Source: CAD feature listing. Evaluate the final solid. Frame: model axes, mm. A direction names the side the tool comes from. Round coordinates to 2 decimals unless told otherwise and drop trailing zeros. Write each loop counter-clockwise with the first axis right and the second up, starting at its lowest first coordinate (ties: lowest second). Pieces come first, ordered by that corner, then holes.
from build123d import *

# Parameters (mm, degrees)
F1_DEPTH    = 2.25
F2_R        = 10.9
F3_DEPTH    = 10.6
F5_DEPTH    = 9.5
F6_T2_ANGLE = 290.6956436441
F6_T4_ANGLE = 110.5630137602
F7_R        = 8.6
F8_DEPTH    = 10
F9_R        = 7.38
F10_DEPTH   = 7
F11_R       = 10.9
F11_R_2     = 9.6734059383
F12_DEPTH   = 8
F13_R       = 9.5
F14_DEPTH   = 1


# Not quite as in the source:
# - a fillet or chamfer that OpenCascade refuses, or shapes differently, is made with other operations: its cross-section is extruded or revolved along the edge and cut away or added


with BuildPart() as f1:
    # F0 (on Top) → F1 (new body)
    with BuildSketch(Plane.XY):
        Polygon((0, 9), (9, 0), (23, 0), (32, 9), (32, 23), (23, 32), (9, 32), (0, 23), align=None)
    extrude(amount=F1_DEPTH)

    # F2 (on Top) → F3 (join)
    with BuildSketch(Plane.XY):
        with Locations((16, 16)):
            Circle(F2_R)
    extrude(amount=F3_DEPTH)

    # F4 (on face) → F5 (join)
    with BuildSketch(Plane(origin=(0, 0, 0), x_dir=(1, 0, 0), z_dir=(0, 0, -1))):
        with BuildLine():
            ThreePointArc((10.8502427242, -6.45), (10.4390813008, -25.3165810908), (26.85, -16))
            ThreePointArc((26.85, -16), (25.3165810908, -10.4390813008), (21.1497572758, -6.45))
            Line((21.1497572758, -6.45), (10.8502427242, -6.45))
        make_face()
    extrude(amount=F5_DEPTH)

    # F6: chamfer of 1.5 on 2 edges, made by hand

    # F6_s1 → F6_t2 (revolve, cut)
    with BuildSketch(Plane(origin=(19.2912753227, 7.2878893438, 0), x_dir=(0, 0, 1), z_dir=(0.9354709038, 0.3534037184, 0))):
        with BuildLine():
            Line((-7.9575735931, 1.5793514401), (-9.5424264069, -0.0055013736))
            Line((-9.5424264069, -0.0055013736), (-9.5724264069, -0.0055013736))
            ThreePointArc((-9.5724264069, -0.0055013736), (-9.53, 0.7657118298), (-9.53, 1.5369250333))
            Line((-9.53, 1.5369250333), (-9.5, 1.5669250333))
            ThreePointArc((-9.5, 1.5669250333), (-8.7287867966, 1.5669250333), (-7.9575735931, 1.6093514401))
            Line((-7.9575735931, 1.6093514401), (-7.9575735931, 1.5793514401))
        make_face()
    revolve(axis=Axis((16, 16, -9.5), (0, 0, -1)), revolution_arc=F6_T2_ANGLE, mode=Mode.SUBTRACT)

    # F6_s3 → F6_t4 (revolve, cut)
    with BuildSketch(Plane.XZ.offset(-16)):
        with BuildLine():
            Line((26.8924264069, -7.9575735931), (25.3075735931, -9.5424264069))
            Line((25.3075735931, -9.5424264069), (25.3075735931, -9.5724264069))
            ThreePointArc((25.3075735931, -9.5724264069), (26.0787867966, -9.53), (26.85, -9.53))
            Line((26.85, -9.53), (26.88, -9.5))
            ThreePointArc((26.88, -9.5), (26.88, -8.7287867966), (26.9224264069, -7.9575735931))
            Line((26.9224264069, -7.9575735931), (26.8924264069, -7.9575735931))
        make_face()
    revolve(axis=Axis((16, 16, -9.5), (0, 0, -1)), revolution_arc=F6_T4_ANGLE, mode=Mode.SUBTRACT)

    # F7 (on face) → F8 (join)
    with BuildSketch(Plane(origin=(0, 0, -9.5), x_dir=(1, 0, 0), z_dir=(0, 0, -1))):
        with Locations((16, -16)):
            Circle(F7_R)
    extrude(amount=F8_DEPTH)

    # F9 (on face) → F10 (cut)
    with BuildSketch(Plane.XY.offset(10.6)):
        with Locations((16, 16)):
            Circle(F9_R)
    extrude(amount=-F10_DEPTH, mode=Mode.SUBTRACT)

    # F11 (on face) → F12 (cut)
    with BuildSketch(Plane.XY.offset(10.6)):
        with Locations((16, 16)):
            Circle(F11_R)
        with Locations((16, 16)):
            Circle(F11_R_2, mode=Mode.SUBTRACT)
    extrude(amount=-F12_DEPTH, mode=Mode.SUBTRACT)

    # F13 (on face) → F14 (cut)
    with BuildSketch(Plane(origin=(0, 0, -19.5), x_dir=(1, 0, 0), z_dir=(0, 0, -1))):
        with Locations((16, -16)):
            Circle(F13_R)
    extrude(amount=-F14_DEPTH, mode=Mode.SUBTRACT)


solid = f1.part
1) Contact query for flat-ended pins moving along their axis: P1, Ø2, axis at x = 12, y = 12.5, coming from the +Z side; P2, Ø3, axis at x = 9.5, z = -14.5, coming from the -Y side; P3, Ø5, axis at x = 3.5, z = 1, coming from the +Y side. Output: stop coordinate, or through.
Taken from the geometry:
P1: stops at z = 3.6
P2: stops at y = 9
P3: stops at y = 29
2) Section query D-D on z = -2.75. Return the cut outline in (x, y).
Taken from the geometry:
outline: (10.85, 6.45) - (21.15, 6.45) arc R10.85 ccw (long way) to start
3) Reachability of faces 1 (the face through (7.35, 9.37, 2.42)), 2 (the face through (16, 6, 0)), 3 (the face through (16, 16, -18.5)) from +Z, -Z, +X, -X, +Y, -Y: full face, straight path, thin tool, end or side. Return the list, or none.
Taken from the geometry:
face 1: +Z
face 2: -Z
face 3: -Z, +X, -X, +Y, -Y
4) Material intervals for line 1 (Y direction, x = 16, z = 8); line 2 (Z direction, x = 23.5, y = 29); line 3 (X direction, y = 20, z = 6), sorted ascending.
Taken from the geometry:
line 1: y = 6.33 to 8.62, 23.38 to 25.67
line 2: z = 0 to 2.25
line 3: x = 7.19 to 9.8, 22.2 to 24.81
5) Section query C-C on y = 30. Return the cut outline in (x, z), then the cut area to 3 significant figures.
Taken from the geometry:
outline: (7, 0) - (25, 0) - (25, 2.25) - (7, 2.25) - close
area: 40.5 mm2
6) Section query A-A on x = 16. Return the cut outline in (y, z).
Taken from the geometry:
outline: (0, 0) - (6.45, 0) - (6.45, -9.3) - (6.65, -9.5) - (7.4, -9.5) - (7.4, -18.5) - (24.6, -18.5) - (24.6, -9.5) - (25.35, -9.5) - (26.85, -8) - (26.85, 0) - (32, 0) - (32, 2.25) - (26.9, 2.25) - (26.9, 2.6) - (25.67, 2.6) - (25.67, 10.6) - (23.38, 10.6) - (23.38, 3.6) - (8.62, 3.6) - (8.62, 10.6) - (6.33, 10.6) - (6.33, 2.6) - (5.1, 2.6) - (5.1, 2.25) - (0, 2.25) - close
7) Pull-direction query (X, two-part tool) for faces 4 (the face through (16, 6.45, -5)), 5 (the face through (0, 16, 1)), 6 (the face through (14.4, 8.795, 7.149)); classes: released by +X, released by -X, zero draft, split by the parting line, or undercut.
Taken from the geometry:
face 4: zero draft
face 5: released by -X
face 6: undercut
8) Section query B-B on z = 4.5. Return the cut outline in (x, y).
Taken from the geometry:
outline: circle Ø19.35 at (16, 16); hole circle Ø14.76 at (16, 16)
